```python
from build123d import *

# Parameters (mm, degrees)
SKETCH_1_W          = 68
SKETCH_1_H          = 30
EXTRUDE_1_DEPTH     = 3
SKETCH_2_R          = 3
EXTRUDE_2_DEPTH     = 2
EXTRUDE_START       = -28
SKETCH_2_2_R        = 3
EXTRUDE_3_DEPTH     = 2
SKETCH_3_R          = 3.5
CUT_EXTRUDE_1_DEPTH = 12


with BuildPart() as part:
    # 草图1 → 凸台-拉伸1 (new body)
    with BuildSketch(Plane(origin=(0, 0, 0), x_dir=(1, 0, 0), z_dir=(0, 1, 0))):
        with Locations((34, 15)):
            Rectangle(SKETCH_1_W, SKETCH_1_H)
    extrude(amount=EXTRUDE_1_DEPTH)

    # 草图2 → 凸台-拉伸2 (add)
    with BuildSketch(Plane.XY):
        with BuildLine():
            Line((15, 3), (26.450876235, 35.647778385))
            ThreePointArc((26.450876235, 35.647778385), (34, 41), (41.549123765, 35.647778385))
            Line((41.549123765, 35.647778385), (53, 3))
            Line((53, 3), (15, 3))
        make_face()
        with Locations((34, 33)):
            Circle(SKETCH_2_R, mode=Mode.SUBTRACT)
    extrude(amount=-EXTRUDE_2_DEPTH)

    # 草图2<2> → 凸台-拉伸3 (add)
    with BuildSketch(Plane.XY.offset(EXTRUDE_START)):
        with BuildLine():
            Line((15, 3), (26.450876235, 35.647778385))
            ThreePointArc((26.450876235, 35.647778385), (34, 41), (41.549123765, 35.647778385))
            Line((41.549123765, 35.647778385), (53, 3))
            Line((53, 3), (15, 3))
        make_face()
        with Locations((34, 33)):
            Circle(SKETCH_2_2_R, mode=Mode.SUBTRACT)
    extrude(amount=-EXTRUDE_3_DEPTH)

    # 草图3 → 切除-拉伸1 (cut)
    with BuildSketch(Plane.XZ):
        with Locations(Location((6, -7, 0), (0, 0, 270))):
            Circle(SKETCH_3_R)
        with Locations(Location((6, -23, 0), (0, 0, 270))):
            Circle(SKETCH_3_R)
        with Locations(Location((62, -7, 0), (0, 0, 270))):
            Circle(SKETCH_3_R)
        with Locations(Location((62, -23, 0), (0, 0, 270))):
            Circle(SKETCH_3_R)
    extrude(amount=-CUT_EXTRUDE_1_DEPTH, mode=Mode.SUBTRACT)


solid = part.part
```
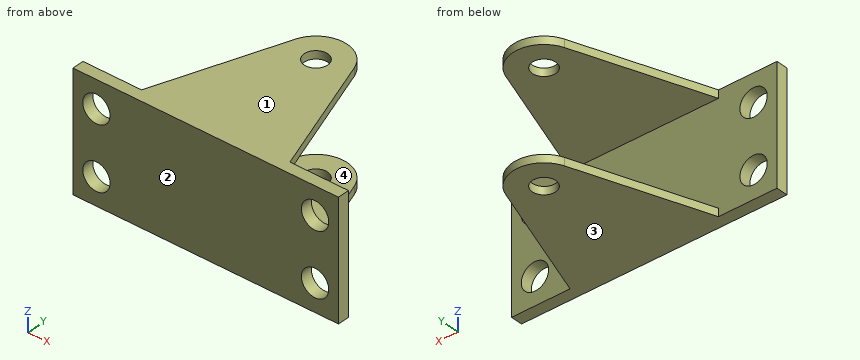
The listing builds one solid part. Answer for the finished solid, in the listing's coordinates (mm). Face numbers are marked on the shaded views. Coordinates: 2 decimals unless noted, no trailing zeros. Loops run counter-clockwise (first coordinate to the right, second up) from the corner with the lowest first, then second, coordinate; pieces in that order, holes last. Notation, with made-up numbers: M 89,-23 L 95,-23 A23 ccw 95,-5 Z; hole C 52.5,14.5 d10. An arc over 180 degrees is marked long. Answer as a JSON object with one key per item and string values. Group by question number.
Item 1: This flat-tipped pin is pushed along its axis until it touches: P1, Ø8, axis at x = 62, z = -23, coming from the +Y side. Where does it stop, or does it pass through?
Item 2: Section B-B (x = 34) is taken. Write down the section's boundary in (y, z).
Item 3: Consider L1, parallel to X at y = 1.5, z = -23; L2, parallel to Z at x = 45, y = 12.5; L3, parallel to Y at x = 30.5, z = -13. Determine where each line is inside the solid, lowest interval first.
Item 4: Determine the mould class of the marked faces 1, 2, 3 and 4 for opening direction Z: +Z half, -Z half, draft (parallel to the pull), parting line (faces both ways), or undercut.
Item 5: Section C-C (y = 33) is taken. Write down the section's boundary in (x, z), and give its area (3 significant figures).
Item 6: Section D-D (y = 27) is taken. Write down the section's boundary in (x, z).
Item 7: Section A-A (z = -23) is taken. Write down the section's boundary in (x, y).
Solved:
{
 "1": {"P1": "stops at y = 3"},
 "2": {"outline": "M 0,-30 L 30,-30 L 30,-28 L 3,-28 L 3,-2 L 30,-2 L 30,0 L 0,0 Z; M 36,-30 L 41,-30 L 41,-28 L 36,-28 Z; M 36,-2 L 41,-2 L 41,0 L 36,0 Z"},
 "3": {"L1": "x = 0 to 2.5, 9.5 to 58.5, 65.5 to 68", "L2": "z = -30 to -28, -2 to 0", "L3": "y = 0 to 3"},
 "4": {"face 1": "+Z half", "face 2": "draft", "face 3": "-Z half", "face 4": "undercut"},
 "5": {"outline": "M 25.52,-30 L 31,-30 L 31,-28 L 25.52,-28 Z; M 25.52,-2 L 31,-2 L 31,0 L 25.52,0 Z; M 37,-30 L 42.48,-30 L 42.48,-28 L 37,-28 Z; M 37,-2 L 42.48,-2 L 42.48,0 L 37,0 Z", "area": "43.8 mm2"},
 "6": {"outline": "M 23.42,-30 L 44.58,-30 L 44.58,-28 L 23.42,-28 Z; M 23.42,-2 L 44.58,-2 L 44.58,0 L 23.42,0 Z"},
 "7": {"outline": "M 0,0 L 2.5,0 L 2.5,3 L 0,3 Z; M 9.5,0 L 58.5,0 L 58.5,3 L 9.5,3 Z; M 65.5,0 L 68,0 L 68,3 L 65.5,3 Z"}
}
